Source: CAD feature listing. Evaluate the final solid. Frame: model axes, mm. Face numbers are marked on the shaded views. A direction names the side the tool comes from. Coordinates: 2 decimals unless noted, no trailing zeros. Write each loop counter-clockwise with the first axis right and the second up, starting at its lowest first coordinate (ties: lowest second). Pieces come first, ordered by that corner, then holes. Notation, with made-up numbers: M 61,30 L 104,30 A23 cw 104,43 Z; hole C -33,46.5 d7. An arc over 180 degrees is marked long. One line per item, written item: value. Start each with the question number.
Item 1: Cut plane A-A, the plane z = -16. Output: boundary loops of the cut face in (x, y), then the cut area to 3 significant figures.
Item 2: Cut plane D-D, the plane z = -14.5. Output: boundary loops of the cut face in (x, y).
Item 3: Ray query, L1, parallel to X at y = -2.55, z = -16; L2, parallel to X at y = -1.1, z = -16; L3, parallel to Z at x = 26, y = -2.55. Return the intervals inside material, ascending. Write a range as from..to.
Item 4: Pin query (flat end, axial travel): P1, Ø2, axis at y = -1, z = -18.5, coming from the +X side; P2, Ø3.5, axis at x = 9, z = -16, coming from the -Y side. Return the tip coordinate at first contact, or that it passes through.
Item 5: Set-up query: the marked faces 4, 5 and 6. Return all of +Z, -Z, +X, -X, +Y, -Y with unobstructed straight access to the full face (end or side cutting, diameter ignored); none if empty.
Item 6: Cut plane B-B, the plane y = -0.85. Output: boundary loops of the cut face in (x, z), then the cut area to 3 significant figures.
Item 7: Cut plane C-C, the plane x = 9. Output: boundary loops of the cut face in (y, z), then the cut area to 3 significant figures.
Item 8: Mould query, pull axis Z, two halves, no side actions, for the marked faces 1, 2 and 3. Classes: released by +Z, released by -Z, zero draft, split by the parting line, or undercut.
```python
from build123d import *

# Parameters (mm, degrees)
SKETCH_1_W           = 35
SKETCH_1_H           = 20
EXTRUDE_1_DEPTH      = 4
SKETCH_3_W           = 29
SKETCH_3_H           = 7.2
CUT_EXTRUDE_4_DEPTH  = 5
SKETCH_4_W           = 6
SKETCH_4_H           = 6
CUT_EXTRUDE_5_DEPTH  = 5
SKETCH_5_R           = 1.2
CUT_EXTRUDE_6_DEPTH  = 41.509258201
SKETCH_6_R           = 2.2
CUT_EXTRUDE_7_DEPTH  = 2
CUT_EXTRUDE_START    = 4
SKETCH_7_R           = 2.2
CUT_EXTRUDE_8_DEPTH  = 2
SKETCH_8_W           = 40.267995894
SKETCH_8_H           = 24.754572762
CUT_EXTRUDE_9_DEPTH  = 41.509258201
SKETCH_11_W          = 6
SKETCH_11_H          = 20
CUT_EXTRUDE_11_DEPTH = 41.509258201


with BuildPart() as part:
    # 草圖1 → 填料-伸長1 (new body)
    with BuildSketch(Plane(origin=(0, 0, 0), x_dir=(1, 0, 0), z_dir=(0, 1, 0))):
        with Locations((17.5, 10)):
            Rectangle(SKETCH_1_W, SKETCH_1_H)
    extrude_1 = extrude(amount=EXTRUDE_1_DEPTH)

    # 草圖3 → 除料-伸長4 (cut)
    with BuildSketch(Plane(origin=(0, 0, 0), x_dir=(1, 0, 0), z_dir=(0, 1, 0))):
        with Locations((20.5, 3.6)):
            Rectangle(SKETCH_3_W, SKETCH_3_H)
    cut_extrude_4 = extrude(amount=CUT_EXTRUDE_4_DEPTH, mode=Mode.SUBTRACT)

    # 草圖4 → 除料-伸長5 (cut)
    with BuildSketch(Plane(origin=(0, 0, 0), x_dir=(1, 0, 0), z_dir=(0, 1, 0))):
        with Locations((32, 17)):
            Rectangle(SKETCH_4_W, SKETCH_4_H)
    cut_extrude_5 = extrude(amount=CUT_EXTRUDE_5_DEPTH, mode=Mode.SUBTRACT)

    # 草圖5 → 除料-伸長6 (cut, through all)
    with BuildSketch(Plane(origin=(0, 0, 0), x_dir=(1, 0, 0), z_dir=(0, 1, 0))):
        with Locations(Location((3, 16, 0), (0, 0, 270))):
            Circle(SKETCH_5_R)
        with Locations(Location((3, 4, 0), (0, 0, 270))):
            Circle(SKETCH_5_R)
        with Locations(Location((9, 16, 0), (0, 0, 270))):
            Circle(SKETCH_5_R)
        with Locations(Location((26, 16, 0), (0, 0, 270))):
            Circle(SKETCH_5_R)
    cut_extrude_6 = extrude(amount=CUT_EXTRUDE_6_DEPTH, mode=Mode.SUBTRACT)

    # 草圖6 → 除料-伸長7 (cut)
    with BuildSketch(Plane(origin=(0, 0, 0), x_dir=(1, 0, 0), z_dir=(0, 1, 0))):
        with Locations(Location((3, 16, 0), (0, 0, 270))):
            Circle(SKETCH_6_R)
        with Locations(Location((3, 4, 0), (0, 0, 270))):
            Circle(SKETCH_6_R)
    cut_extrude_7 = extrude(amount=CUT_EXTRUDE_7_DEPTH, mode=Mode.SUBTRACT)

    # 草圖7 → 除料-伸長8 (cut)
    with BuildSketch(Plane(origin=(0, 0, 0), x_dir=(1, 0, 0), z_dir=(0, 1, 0)).offset(CUT_EXTRUDE_START)):
        with Locations(Location((9, 16, 0), (0, 0, 90))):
            Circle(SKETCH_7_R)
        with Locations(Location((26, 16, 0), (0, 0, 90))):
            Circle(SKETCH_7_R)
    cut_extrude_8 = extrude(amount=-CUT_EXTRUDE_8_DEPTH, mode=Mode.SUBTRACT)

    # 鏡射1: 填料-伸長1, 除料-伸長4, 除料-伸長5, 除料-伸長6, 除料-伸長7, 除料-伸長8 across plane
    add(extrude_1.mirror(Plane.ZX))
    add(cut_extrude_4.mirror(Plane.ZX), mode=Mode.SUBTRACT)
    add(cut_extrude_5.mirror(Plane.ZX), mode=Mode.SUBTRACT)
    add(cut_extrude_6.mirror(Plane.ZX), mode=Mode.SUBTRACT)
    add(cut_extrude_7.mirror(Plane.ZX), mode=Mode.SUBTRACT)
    add(cut_extrude_8.mirror(Plane.ZX), mode=Mode.SUBTRACT)

    # 草圖8 → 除料-伸長9 (cut, through all)
    with BuildSketch(Plane(origin=(0, 0, 0), x_dir=(1, 0, 0), z_dir=(0, 1, 0))):
        with Locations((18.825302285, 8.624835494)):
            Rectangle(SKETCH_8_W, SKETCH_8_H)
    extrude(amount=CUT_EXTRUDE_9_DEPTH, mode=Mode.SUBTRACT)

    # 草圖11 → 除料-伸長11 (cut, through all)
    with BuildSketch(Plane(origin=(0, 0, 0), x_dir=(1, 0, 0), z_dir=(0, 1, 0))):
        with Locations((3, 10)):
            Rectangle(SKETCH_11_W, SKETCH_11_H)
    extrude(amount=-CUT_EXTRUDE_11_DEPTH, mode=Mode.SUBTRACT)


solid = part.part
```
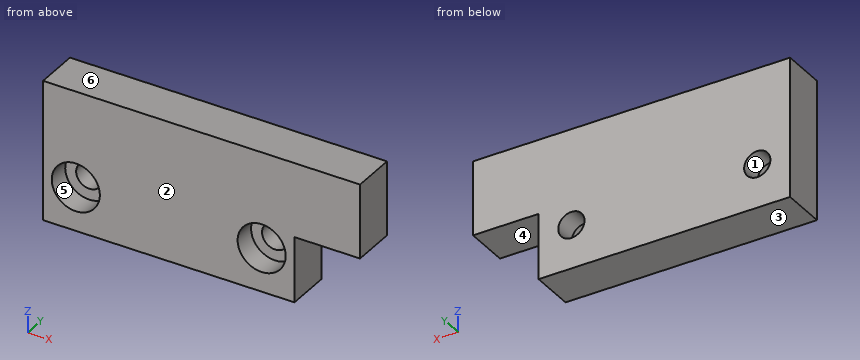
From the geometry:
1. outline: M 6,-4 L 6.8,-4 L 6.8,-2 L 7.8,-2 L 7.8,0 L 6,0 Z; M 10.2,-2 L 11.2,-2 L 11.2,-4 L 23.8,-4 L 23.8,-2 L 24.8,-2 L 24.8,0 L 10.2,0 Z; M 27.2,-2 L 28.2,-2 L 28.2,-4 L 29,-4 L 29,0 L 27.2,0 Z
1. area: 64.8 mm²
2. outline: M 6,-4 L 7.39,-4 L 7.39,-2 L 10.61,-2 L 10.61,-4 L 24.39,-4 L 24.39,-2 L 27.61,-2 L 27.61,-4 L 29,-4 L 29,0 L 6,0 Z
3. L1: x = 6..6.8, 11.2..23.8, 28.2..29
3. L2: x = 6..7.8, 10.2..24.8, 27.2..29
3. L3: z = -20..-18.2, -13.8..-7.2
4. P1: stops at x = 29
4. P2: stops at y = -2
5. face 4: -Z, +X, +Y, -Y
5. face 5: -Y
5. face 6: +Z, +X, -X, +Y, -Y
6. outline: M 6,-20 L 29,-20 L 29,-14 L 35,-14 L 35,-7.2 L 6,-7.2 Z; hole C 9,-16 d2.4; hole C 26,-16 d2.4
6. area: 326 mm²
7. outline: M -4,-20 L 0,-20 L 0,-17.2 L -2,-17.2 L -2,-18.2 L -4,-18.2 Z; M -4,-13.8 L -2,-13.8 L -2,-14.8 L 0,-14.8 L 0,-7.2 L -4,-7.2 Z
7. area: 37.6 mm²
8. face 1: undercut
8. face 2: zero draft
8. face 3: released by -Z
